```python
from build123d import *

# Parameters (mm, degrees)
BOSS_EXTRUDE1_DEPTH = 15
SKETCH5_R           = 2.5
CUT_EXTRUDE1_DEPTH  = 10


with BuildPart() as part:
    # Sketch1 → Boss-Extrude1 (new body)
    with BuildSketch(Plane(origin=(0, 0, 0), x_dir=(1, 0, 0), z_dir=(0, 1, 0))):
        with BuildLine():
            Line((0, 22.856339564), (0, -22.143660436))
            Line((0, -22.143660436), (10, -22.143660436))
            Line((10, -22.143660436), (10, -12.143660436))
            Line((10, -12.143660436), (35, -12.143660436))
            Line((35, -12.143660436), (35, -3.143660436))
            Line((35, -3.143660436), (23.095240671, -3.143660436))
            ThreePointArc((23.095240671, -3.143660436), (14.232337293, -0.501428414), (22.389683957, 3.856339564))
            Line((22.389683957, 3.856339564), (35, 3.856339564))
            Line((35, 3.856339564), (35, 12.856339564))
            Line((35, 12.856339564), (10, 12.856339564))
            Line((10, 12.856339564), (10, 22.856339564))
            Line((10, 22.856339564), (0, 22.856339564))
        make_face()
    extrude(amount=BOSS_EXTRUDE1_DEPTH)

    # Sketch5 → Cut-Extrude1 (cut)
    with BuildSketch(Plane(origin=(10, 0, 0), x_dir=(0, 0, -1), z_dir=(1, 0, 0))):
        with Locations((-17.085223361, 7.697334505)):
            Circle(SKETCH5_R)
        with Locations((17.783324683, 7.697334505)):
            Circle(SKETCH5_R)
    extrude(amount=-CUT_EXTRUDE1_DEPTH, mode=Mode.SUBTRACT)


solid = part.part
```
The model under review builds one solid part; all positions refer to its coordinate system, in mm. A direction names the side the tool comes from. Give positions to 0.01 mm unless a question says otherwise; leave off trailing zeros. Write each loop counter-clockwise with the first axis right and the second up, starting at its lowest first coordinate (ties: lowest second). Pieces come first, ordered by that corner, then holes. Notation, with made-up numbers: (-5, -37) - (6, -37) arc R18 ccw to (6, -28) - close; hole circle Ø6 at (4.25, 65). An arc over 180 degrees is marked (long way). Answer in a Markdown table with one row per item. Add a question column.
1. Tool access review of faces 5 (the flat face through (10, 5.7, 19.4)), 6 (the flat face through (10, 6, -20)), 7 (the flat face through (29, 7, 3.144)): name each direction out of +Z, -Z, +X, -X, +Y, -Y from which nothing blocks a thin tool from reaching the whole face with its end or side.
2. We need section D-D on z = 0. Write out the cut boundary in (x, y).
3. We need section A-A on x = 24. Write out the cut boundary in (y, z), then the cut area to 3 significant figures.
4. Draft analysis for pull direction Y (two halves, no side actions). For faces 1 (the cylindrical face through (5.07, 10.176, 17.411)), 2 (the flat face through (13, 0, -1)), 3 (the cylindrical face through (5.07, 9.805, -19.127)), 4 (the flat face through (35, 7, -8)), state which applies: +Y half, -Y half, draft (parallel to the pull), parting line (faces both ways), or undercut.
5. We need section C-C on x = 7. Write out the cut boundary in (y, z), then the cut area to 3 significant figures.
6. We need section B-B on z = -16.5. Write out the cut boundary in (x, y), then the cut area to 3 significant figures.
7. Insertion check: P1, Ø5, axis at y = 5, z = -16.5, coming from the +X side; P2, Ø6, axis at x = 31.5, z = -16, coming from the +Y side; P3, Ø1, axis at x = 18, y = 5, coming from the +Z side. Each pin has a flat end and moves straight along its axis. Give the tip position at first contact, or say it passes through.
8. Wall thickness on line 1 along Z through (x, y) = (27, 10.25); line 2 along Z through (x, y) = (19, 4.25); line 3 along Z through (x, y) = (11, 8.25): over which ranges is each line inside the solid? List them lowest first. Write a range as [from, to].
Ans:
| question | item | result |
|---|---|---|
| 1 | face 5 | +Z, +X, +Y, -Y |
| 1 | face 6 | -Z, +X, +Y, -Y |
| 1 | face 7 | +X, +Y, -Y |
| 2 | outline | (0, 0) - (14.21, 0) - (14.21, 15) - (0, 15) - close |
| 3 | outline | (0, -12.86) - (15, -12.86) - (15, -3.86) - (0, -3.86) - close; (0, 3.14) - (15, 3.14) - (15, 12.14) - (0, 12.14) - close |
| 3 | area | 270 mm^2 |
| 4 | face 1 | undercut |
| 4 | face 2 | -Y half |
| 4 | face 3 | undercut |
| 4 | face 4 | draft |
| 5 | outline | (0, -22.86) - (15, -22.86) - (15, 22.14) - (0, 22.14) - close; hole circle Ø5 at (7.7, -17.78); hole circle Ø5 at (7.7, 17.09) |
| 5 | area | 636 mm^2 |
| 6 | outline | (0, 0) - (10, 0) - (10, 5.55) - (0, 5.55) - close; (0, 9.84) - (10, 9.84) - (10, 15) - (0, 15) - close |
| 6 | area | 107 mm^2 |
| 7 | P1 | stops at x = 10 |
| 7 | P2 | passes through |
| 7 | P3 | stops at z = 12.14 |
| 8 | line 1 | z = [-12.86, -3.86], [3.14, 12.14] |
| 8 | line 2 | z = [-12.86, -5], [5, 12.14] |
| 8 | line 3 | z = [-12.86, 12.14] |
